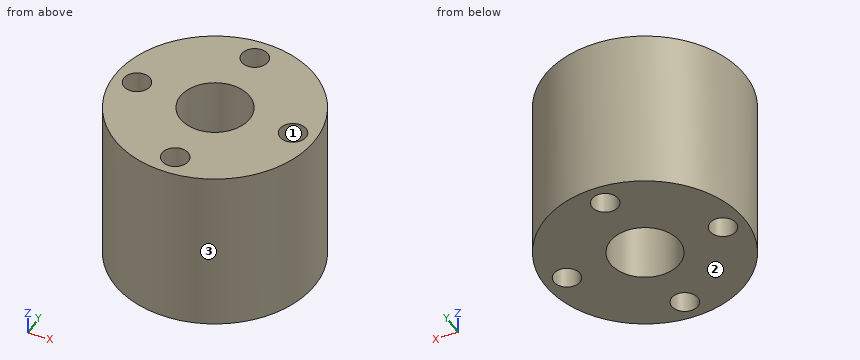
from build123d import *

# Parameters (mm, degrees)
SKETCH1_R             = 11.43
SKETCH1_R_2           = 3.96875
BOSS_EXTRUDE1_DEPTH   = 19.05
F_3_0MM_DOWEL_HOLE1_D = 3
CIRPATTERN1_COUNT     = 4


with BuildPart() as part:
    # Sketch1 → Boss-Extrude1 (new body)
    with BuildSketch(Plane.XY):
        with Locations(Location((0, 0, 0), (0, 0, 180))):
            Circle(SKETCH1_R)
        with Locations(Location((0, 0, 0), (0, 0, 180))):
            Circle(SKETCH1_R_2, mode=Mode.SUBTRACT)
    extrude(amount=BOSS_EXTRUDE1_DEPTH)

    # Ø3.0mm Dowel Hole1 (through all)
    with Locations(Plane.XY.offset(19.05)):
        with Locations((0, 8.89)):
            f_3_0mm_dowel_hole1 = Hole(F_3_0MM_DOWEL_HOLE1_D / 2)

    # CirPattern1: Ø3.0mm Dowel Hole1 ×4 about axis
    cirpattern1_axis = Axis((0, 0, 0), (0, 0, 1))
    for i in range(1, CIRPATTERN1_COUNT):
        add(f_3_0mm_dowel_hole1.rotate(cirpattern1_axis, i * 360 / CIRPATTERN1_COUNT), mode=Mode.SUBTRACT)


solid = part.part
Read the model definition and answer for the solid it produces. Units are mm, in the model's axes. Face numbers are marked on the shaded views. Round coordinates to 2 decimals unless told otherwise and drop trailing zeros. Write each loop counter-clockwise with the first axis right and the second up, starting at its lowest first coordinate (ties: lowest second). Pieces come first, ordered by that corner, then holes.
Q1. Find section A-A on x = 0. Determine the outline of the cut face in (y, z), and give its area (3 significant figures).
Values:
outline: (-11.43, 0) - (-10.39, 0) - (-10.39, 19.05) - (-11.43, 19.05) - close; (-7.39, 0) - (-3.97, 0) - (-3.97, 19.05) - (-7.39, 19.05) - close; (3.97, 0) - (7.39, 0) - (7.39, 19.05) - (3.97, 19.05) - close; (10.39, 0) - (11.43, 0) - (11.43, 19.05) - (10.39, 19.05) - close
area: 170 mm2
Q2. The mould has two halves that part along X. Classify the marked faces 1, 2 and 3: released by +X, released by -X, zero draft, split by the parting line, or undercut.
Values:
face 1: undercut
face 2: zero draft
face 3: split by the parting line
Q3. Find section D-D on z = 5.5. Determine the outline of the cut face in (x, y).
Values:
outline: circle Ø22.86 at (0, 0); hole circle Ø3 at (-8.89, 0); hole circle Ø7.94 at (0, 0); hole circle Ø3 at (0, -8.89); hole circle Ø3 at (0, 8.89); hole circle Ø3 at (8.89, 0)
Q4. Find section C-C on x = -8. Determine the outline of the cut face in (y, z), and give its area (3 significant figures).
Values:
outline: (-8.16, 0) - (-1.21, 0) - (-1.21, 19.05) - (-8.16, 19.05) - close; (1.21, 0) - (8.16, 0) - (8.16, 19.05) - (1.21, 19.05) - close
area: 265 mm2
Q5. Flat-ended cylindrical pins translate along their axes: P1, Ø5, axis at y = -6, z = 14.5, coming from the -X side; P2, Ø4, axis at x = -9, z = 6.5, coming from the -Y side; P3, Ø4, axis at x = 8.89, y = 0, coming from the -Z side; P4, Ø6, axis at x = -4.5, z = 16.5, coming from the +Y side. Find the tip coordinate at first contact, or state that the pin passes through.
Values:
P1: stops at x = -10.88
P2: stops at y = -9.04
P3: stops at z = 0
P4: stops at y = 11.33
Q6. Straight lines are drawn through the part: line 1 (Y direction, x = 0, z = 15); line 2 (X direction, y = -1.25, z = 16.5); line 3 (X direction, y = -2.75, z = 15.25). For each, find the intervals that lie inside material, in ascending order.
Values:
line 1: y = -11.43 to -10.39, -7.39 to -3.97, 3.97 to 7.39, 10.39 to 11.43
line 2: x = -11.36 to -9.72, -8.06 to -3.77, 3.77 to 8.06, 9.72 to 11.36
line 3: x = -11.09 to -2.86, 2.86 to 11.09
Q7. Find section B-B on y = 3. Determine the outline of the cut face in (x, z).
Values:
outline: (-11.03, 0) - (-2.6, 0) - (-2.6, 19.05) - (-11.03, 19.05) - close; (2.6, 0) - (11.03, 0) - (11.03, 19.05) - (2.6, 19.05) - close
